Source: CAD feature listing. Evaluate the final solid. Frame: model axes, mm. A direction names the side the tool comes from. Round coordinates to 2 decimals unless told otherwise and drop trailing zeros. Order: outer loops, then holes, each group sorted by start corner. A loop starts at its lowest first (then second) coordinate and runs counter-clockwise, first axis right, second up. Notation, with made-up numbers: (65.25, 64) -> (115.25, 64) arc R12 cw to (115.25, 68) -> close; hole circle Ø8 at (53, 85). An arc over 180 degrees is marked (long way). Write item = value, one per line. Start each with the question number.
(1) Draft query along Y for faces 5 (the face through (-9.35, 22.42, 15.97)), 6 (the face through (10.35, 13, 9)), 7 (the face through (0, 0, 9)), 8 (the face through (11.62, 16, 9)). Return one class per face: released by +Y, released by -Y, zero draft, split by the parting line, or undercut.
(2) Ray query, line 1 (X direction, y = 22, z = 7); line 2 (X direction, y = 2.5, z = 7.5); line 3 (Y direction, x = 2.5, z = 12.75). Return the intervals inside material, ascending.
(3) Cut plane A-A on y = 3.5. Return the cut outline in (x, z).
(4) Reachability of faces 1 (the face through (10.35, 35, 18)), 2 (the face through (9.35, 22.13, 15.68)), 3 (the face through (-8.318, 26, 12)), 4 (the face through (0, 1.27, 9)) from +Z, -Z, +X, -X, +Y, -Y: full face, straight path, thin tool, end or side. Return the list, or none.
(5) Cut plane B-B on z = 17.25. Return the cut outline in (x, y).
(6) Cut plane D-D on y = 25.5. Return the cut outline in (x, z), then the cut area to 3 significant figures.
(7) Cut plane C-C on x = -9. Return the cut outline in (y, z).
(8) Contact query for flat-ended pins moving along their axis: pin 1 Ø8 at (x, z) = (-9, 5.5) entering from +Y; pin 2 Ø2 at (x, y) = (8.5, 14.5) entering from +Z; pin 3 Ø1.5 at (x, y) = (-9, 19.5) entering from -Z; pin 4 Ø5.5 at (x, z) = (3.5, 6.5) entering from +Y. Output: stop coordinate, or through.
from build123d import *

# Parameters (mm, degrees)
F1_DEPTH = 18.542
F3_DEPTH = 23.242
F5_DEPTH = 2.032
F7_DEPTH = 2.032


with BuildPart() as f1:
    # F0 (on Top) → F1 (new body)
    with BuildSketch(Plane.XY):
        with BuildLine():
            Line((-10.3505, 38.1), (-11.6205, 38.1))
            Line((-11.6205, 38.1), (-11.6205, 2.032))
            ThreePointArc((-11.6205, 2.032), (-11.025341, 0.595159), (-9.5885, 0))
            Line((-9.5885, 0), (9.5885, 0))
            ThreePointArc((9.5885, 0), (11.025341, 0.595159), (11.6205, 2.032))
            Line((11.6205, 2.032), (11.6205, 38.1))
            Line((11.6205, 38.1), (10.3505, 38.1))
            Line((10.3505, 38.1), (10.3505, 2.032))
            ThreePointArc((10.3505, 2.032), (10.127315, 1.493185), (9.5885, 1.27))
            Line((9.5885, 1.27), (-9.5885, 1.27))
            ThreePointArc((-9.5885, 1.27), (-10.127315, 1.493185), (-10.3505, 2.032))
            Line((-10.3505, 2.032), (-10.3505, 38.1))
        make_face()
    extrude(amount=F1_DEPTH)

    # F2 (on face) → F3 (cut, through all)
    with BuildSketch(Plane.YZ.offset(11.6205)):
        Polygon((38.1, 0), (38.1, 18.542), (19.558, 0), align=None)
    extrude(amount=-F3_DEPTH, mode=Mode.SUBTRACT)

    # F4 (on face) → F5 (join)
    with BuildSketch(Plane.YZ.offset(-10.3505)):
        with BuildLine():
            Line((22.273413, 2.715413), (35.384587, 15.826587))
            ThreePointArc((35.384587, 15.826587), (22.273413, 15.826587), (22.273413, 2.715413))
        make_face()
    extrude(amount=F5_DEPTH)

    # F6 (on face) → F7 (join)
    with BuildSketch(Plane(origin=(10.3505, 0, 0), x_dir=(0, -1, 0), z_dir=(-1, 0, 0))):
        with BuildLine():
            Line((-35.384587, 15.826587), (-22.273413, 2.715413))
            ThreePointArc((-22.273413, 2.715413), (-22.273413, 15.826587), (-35.384587, 15.826587))
        make_face()
    extrude(amount=F7_DEPTH)


solid = f1.part
Evaluation:
q1.face_5 = undercut
q1.face_6 = undercut
q1.face_7 = released by -Y
q1.face_8 = zero draft
q2.line_1 = -11.62 to -8.32, 8.32 to 11.62
q2.line_2 = -11.62 to -10.35, 10.35 to 11.62
q2.line_3 = 0 to 1.27
q3.outline = (-11.62, 0) -> (-10.35, 0) -> (-10.35, 18.54) -> (-11.62, 18.54) -> close; (10.35, 0) -> (11.62, 0) -> (11.62, 18.54) -> (10.35, 18.54) -> close
q4.face_1 = +Z, +Y
q4.face_2 = none
q4.face_3 = +Z, -Z, +Y
q4.face_4 = +Z, -Z
q5.outline = (-11.62, 2.03) arc R2.03 ccw to (-9.59, 0) -> (9.59, 0) arc R2.03 ccw to (11.62, 2.03) -> (11.62, 36.81) -> (10.35, 36.81) -> (10.35, 33.55) -> (8.32, 33.55) -> (8.32, 24.11) -> (10.35, 24.11) -> (10.35, 2.03) arc R0.76 cw to (9.59, 1.27) -> (-9.59, 1.27) arc R0.76 cw to (-10.35, 2.03) -> (-10.35, 24.11) -> (-8.32, 24.11) -> (-8.32, 33.55) -> (-10.35, 33.55) -> (-10.35, 36.81) -> (-11.62, 36.81) -> close
q6.outline = (-11.62, 5.94) -> (-8.32, 5.94) -> (-8.32, 17.92) -> (-10.35, 17.92) -> (-10.35, 18.54) -> (-11.62, 18.54) -> close; (8.32, 5.94) -> (11.62, 5.94) -> (11.62, 18.54) -> (10.35, 18.54) -> (10.35, 17.92) -> (8.32, 17.92) -> close
q6.area = 80.7 mm^2
q7.outline = (0, 0) -> (1.27, 0) -> (1.27, 18.54) -> (0, 18.54) -> close; (22.27, 2.72) -> (35.38, 15.83) arc R9.27 ccw to start
q8.pin_1 = 29.06
q8.pin_2 = through
q8.pin_3 = 5.76
q8.pin_4 = 1.27
